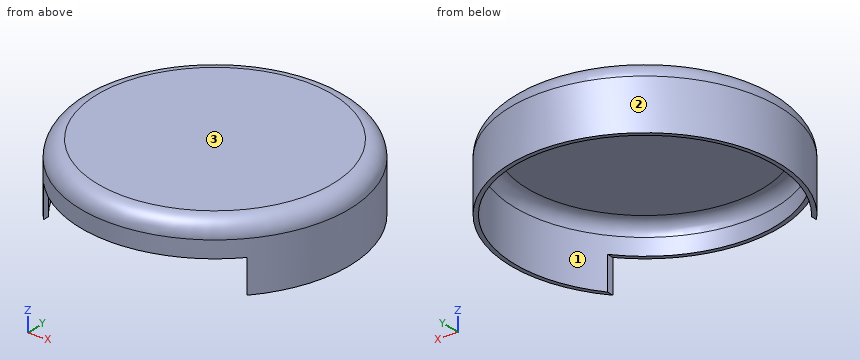
from build123d import *

# Parameters (mm, degrees)
F2_T     = -2.5
F3_W     = 120
F3_H     = 30
F4_DEPTH = 100


with BuildPart() as f1:
    # F0 (on Right) → F1 (revolve)
    with BuildSketch(Plane.YZ):
        with BuildLine():
            Line((-80, -10), (-80, -40))
            Line((-80, -40), (0, -40))
            Line((0, -40), (0, 0))
            Line((0, 0), (-70, 0))
            ThreePointArc((-70, 0), (-77.071068, -2.928932), (-80, -10))
        make_face()
    revolve(axis=Axis((0, 0, -20), (0, 0, -1)))

    # F2
    f2_openings = [f1.faces().sort_by_distance(p)[0] for p in [
        (0, 0, -40),
    ]]
    offset(amount=F2_T, openings=f2_openings)

    # F3 (on Front) → F4 (cut)
    with BuildSketch(Plane.XZ):
        with Locations((0, -35)):
            Rectangle(F3_W, F3_H)
    extrude(amount=F4_DEPTH, mode=Mode.SUBTRACT)


solid = f1.part
The model under review builds one solid part; all positions refer to its coordinate system, in mm. Face numbers are marked on the shaded views. Give positions to 0.01 mm unless a question says otherwise; leave off trailing zeros. Write each loop counter-clockwise with the first axis right and the second up, starting at its lowest first coordinate (ties: lowest second). Pieces come first, ordered by that corner, then holes. Notation, with made-up numbers: M -40,-29 L -14,-29 A28 cw -14,6 Z; hole C 70.5,36.25 d4. An arc over 180 degrees is marked long. One line per question, with ' | ' between items. Start each with the question number.
Item 1: Wall thickness on line 1 (X direction, y = 0, z = -19); line 2 (Z direction, x = 25, y = 19.5); line 3 (X direction, y = 52, z = -24): over which ranges is each line inside the solid? List them lowest first. Write a range as from..to.
Item 2: We need section C-C on z = -25. Write out the cut boundary in (x, y), plus the area to 3 significant figures.
Item 3: We need section B-B on x = 0. Write out the cut boundary in (y, z).
Item 4: For pin 1 (12 mm diameter, centred on x = 1, y = -51.5, fed in from -Z); pin 2 (12 mm diameter, centred on x = -45, z = -12, fed in from +Y); pin 3 (15.5 mm diameter, centred on x = -16, y = -69.5, fed in from -Z), all flat-tipped, find the tip position at first contact; note any pin that passes through.
Item 5: We need section A-A on y = 0. Write out the cut boundary in (x, z), plus the area to 3 significant figures.
Item 6: Draft analysis for pull direction X (two halves, no side actions). For the marked faces 1, 2 and 3, state which applies: released by +X, released by -X, zero draft, split by the parting line, or undercut.
Results found:
1) line 1: x = -80..-77.5, 77.5..80 | line 2: z = -2.5..0 | line 3: x = -60.79..-57.47, 57.47..60.79
2) outline: M -60,-52.92 L -60,-49.05 A77.5 cw long 60,-49.05 L 60,-52.92 A80 ccw long Z | area: 896 mm2
3) outline: M -80,-20 L -77.5,-20 L -77.5,-10 A7.5 cw -70,-2.5 L 70,-2.5 A7.5 cw 77.5,-10 L 77.5,-40 L 80,-40 L 80,-10 A10 ccw 70,0 L -70,0 A10 ccw -80,-10 Z
4) pin 1: stops at z = -2.5 | pin 2: stops at y = 69.85 | pin 3: stops at z = -20
5) outline: M -80,-40 L -77.5,-40 L -77.5,-10 A7.5 cw -70,-2.5 L 70,-2.5 A7.5 cw 77.5,-10 L 77.5,-40 L 80,-40 L 80,-10 A10 ccw 70,0 L -70,0 A10 ccw -80,-10 Z | area: 569 mm2
6) face 1: undercut | face 2: split by the parting line | face 3: zero draft
